from build123d import *

# Parameters (mm, degrees)
SKETCH1_R               = 2.5
EXTRUDE1_DEPTH          = 277.5
CUT_EXTRUDE1_DEPTH      = 556.900170894
CUT_EXTRUDE1_DEPTH_BACK = 556.900170894
SKETCH2_W               = 3.3
SKETCH2_H               = 11.078679656
SKETCH3_W               = 21.963498752
SKETCH3_H               = 21.444138823
CUT_EXTRUDE2_DEPTH      = 20


with BuildPart() as part:
    # Sketch1 → Extrude1 (new, symmetric)
    with BuildSketch(Plane.XY):
        with BuildLine():
            Line((0, 3.9), (-2.010912703, 3.9))
            ThreePointArc((-2.010912703, 3.9), (-2.776279568, 4.052240935), (-3.425126266, 4.485786438))
            Line((-3.425126266, 4.485786438), (-5.539339828, 6.6))
            Line((-5.539339828, 6.6), (-5.539339828, 8.2))
            Line((-5.539339828, 8.2), (-3.1, 8.2))
            Line((-3.1, 8.2), (-3.1, 9.5))
            Line((-3.1, 9.5), (-3.4, 9.5))
            ThreePointArc((-3.4, 9.5), (-3.541421356, 9.558578644), (-3.6, 9.7))
            Line((-3.6, 9.7), (-3.6, 10))
            Line((-3.6, 10), (-8.5, 10))
            Line((-8.5, 10), (-11.5, 10))
            Line((-11.5, 10), (-16.4, 10))
            Line((-16.4, 10), (-16.4, 9.7))
            ThreePointArc((-16.4, 9.7), (-16.458578644, 9.558578644), (-16.6, 9.5))
            Line((-16.6, 9.5), (-16.9, 9.5))
            Line((-16.9, 9.5), (-16.9, 8.2))
            Line((-16.9, 8.2), (-14.460660172, 8.2))
            Line((-14.460660172, 8.2), (-14.460660172, 6.6))
            Line((-14.460660172, 6.6), (-16.574873734, 4.485786438))
            ThreePointArc((-16.574873734, 4.485786438), (-17.223720432, 4.052240935), (-17.989087297, 3.9))
            Line((-17.989087297, 3.9), (-20, 3.9))
            Line((-20, 3.9), (-22.010912703, 3.9))
            ThreePointArc((-22.010912703, 3.9), (-22.776279568, 4.052240935), (-23.425126266, 4.485786438))
            Line((-23.425126266, 4.485786438), (-25.539339828, 6.6))
            Line((-25.539339828, 6.6), (-25.539339828, 8.2))
            Line((-25.539339828, 8.2), (-23.1, 8.2))
            Line((-23.1, 8.2), (-23.1, 9.5))
            Line((-23.1, 9.5), (-23.4, 9.5))
            ThreePointArc((-23.4, 9.5), (-23.541421356, 9.558578644), (-23.6, 9.7))
            Line((-23.6, 9.7), (-23.6, 10))
            Line((-23.6, 10), (-28.5, 10))
            ThreePointArc((-28.5, 10), (-29.560660172, 9.560660172), (-30, 8.5))
            Line((-30, 8.5), (-30, 3.6))
            Line((-30, 3.6), (-29.7, 3.6))
            ThreePointArc((-29.7, 3.6), (-29.558578644, 3.541421356), (-29.5, 3.4))
            Line((-29.5, 3.4), (-29.5, 3.1))
            Line((-29.5, 3.1), (-28.2, 3.1))
            Line((-28.2, 3.1), (-28.2, 5.539339828))
            Line((-28.2, 5.539339828), (-26.6, 5.539339828))
            Line((-26.6, 5.539339828), (-24.485786438, 3.425126266))
            ThreePointArc((-24.485786438, 3.425126266), (-24.052240935, 2.776279568), (-23.9, 2.010912703))
            Line((-23.9, 2.010912703), (-23.9, 0))
            Line((-23.9, 0), (-23.9, -2.010912703))
            ThreePointArc((-23.9, -2.010912703), (-24.052240935, -2.776279568), (-24.485786438, -3.425126266))
            Line((-24.485786438, -3.425126266), (-26.6, -5.539339828))
            Line((-26.6, -5.539339828), (-28.2, -5.539339828))
            Line((-28.2, -5.539339828), (-28.2, -3.1))
            Line((-28.2, -3.1), (-29.5, -3.1))
            Line((-29.5, -3.1), (-29.5, -3.4))
            ThreePointArc((-29.5, -3.4), (-29.558578644, -3.541421356), (-29.7, -3.6))
            Line((-29.7, -3.6), (-30, -3.6))
            Line((-30, -3.6), (-30, -8.5))
            ThreePointArc((-30, -8.5), (-29.560660172, -9.560660172), (-28.5, -10))
            Line((-28.5, -10), (-23.6, -10))
            Line((-23.6, -10), (-23.6, -9.7))
            ThreePointArc((-23.6, -9.7), (-23.541421356, -9.558578644), (-23.4, -9.5))
            Line((-23.4, -9.5), (-23.1, -9.5))
            Line((-23.1, -9.5), (-23.1, -8.2))
            Line((-23.1, -8.2), (-25.539339828, -8.2))
            Line((-25.539339828, -8.2), (-25.539339828, -6.6))
            Line((-25.539339828, -6.6), (-23.425126266, -4.485786438))
            ThreePointArc((-23.425126266, -4.485786438), (-22.776279568, -4.052240935), (-22.010912703, -3.9))
            Line((-22.010912703, -3.9), (-20, -3.9))
            Line((-20, -3.9), (-17.989087297, -3.9))
            ThreePointArc((-17.989087297, -3.9), (-17.223720432, -4.052240935), (-16.574873734, -4.485786438))
            Line((-16.574873734, -4.485786438), (-14.460660172, -6.6))
            Line((-14.460660172, -6.6), (-14.460660172, -8.2))
            Line((-14.460660172, -8.2), (-16.9, -8.2))
            Line((-16.9, -8.2), (-16.9, -9.5))
            Line((-16.9, -9.5), (-16.6, -9.5))
            ThreePointArc((-16.6, -9.5), (-16.458578644, -9.558578644), (-16.4, -9.7))
            Line((-16.4, -9.7), (-16.4, -10))
            Line((-16.4, -10), (-11.5, -10))
            Line((-11.5, -10), (-8.5, -10))
            Line((-8.5, -10), (-3.6, -10))
            Line((-3.6, -10), (-3.6, -9.7))
            ThreePointArc((-3.6, -9.7), (-3.541421356, -9.558578644), (-3.4, -9.5))
            Line((-3.4, -9.5), (-3.1, -9.5))
            Line((-3.1, -9.5), (-3.1, -8.2))
            Line((-3.1, -8.2), (-5.539339828, -8.2))
            Line((-5.539339828, -8.2), (-5.539339828, -6.6))
            Line((-5.539339828, -6.6), (-3.425126266, -4.485786438))
            ThreePointArc((-3.425126266, -4.485786438), (-2.776279568, -4.052240935), (-2.010912703, -3.9))
            Line((-2.010912703, -3.9), (0, -3.9))
            Line((0, -3.9), (2.010912703, -3.9))
            ThreePointArc((2.010912703, -3.9), (2.776279568, -4.052240935), (3.425126266, -4.485786438))
            Line((3.425126266, -4.485786438), (5.539339828, -6.6))
            Line((5.539339828, -6.6), (5.539339828, -8.2))
            Line((5.539339828, -8.2), (3.1, -8.2))
            Line((3.1, -8.2), (3.1, -9.5))
            Line((3.1, -9.5), (3.4, -9.5))
            ThreePointArc((3.4, -9.5), (3.541421356, -9.558578644), (3.6, -9.7))
            Line((3.6, -9.7), (3.6, -10))
            Line((3.6, -10), (8.5, -10))
            ThreePointArc((8.5, -10), (9.560660172, -9.560660172), (10, -8.5))
            Line((10, -8.5), (10, -3.6))
            Line((10, -3.6), (9.7, -3.6))
            ThreePointArc((9.7, -3.6), (9.558578644, -3.541421356), (9.5, -3.4))
            Line((9.5, -3.4), (9.5, -3.1))
            Line((9.5, -3.1), (8.2, -3.1))
            Line((8.2, -3.1), (8.2, -5.539339828))
            Line((8.2, -5.539339828), (6.6, -5.539339828))
            Line((6.6, -5.539339828), (4.485786438, -3.425126266))
            ThreePointArc((4.485786438, -3.425126266), (4.052240935, -2.776279568), (3.9, -2.010912703))
            Line((3.9, -2.010912703), (3.9, 0))
            Line((3.9, 0), (3.9, 2.010912703))
            ThreePointArc((3.9, 2.010912703), (4.052240935, 2.776279568), (4.485786438, 3.425126266))
            Line((4.485786438, 3.425126266), (6.6, 5.539339828))
            Line((6.6, 5.539339828), (8.2, 5.539339828))
            Line((8.2, 5.539339828), (8.2, 3.1))
            Line((8.2, 3.1), (9.5, 3.1))
            Line((9.5, 3.1), (9.5, 3.4))
            ThreePointArc((9.5, 3.4), (9.558578644, 3.541421356), (9.7, 3.6))
            Line((9.7, 3.6), (10, 3.6))
            Line((10, 3.6), (10, 8.5))
            ThreePointArc((10, 8.5), (9.560660172, 9.560660172), (8.5, 10))
            Line((8.5, 10), (3.6, 10))
            Line((3.6, 10), (3.6, 9.7))
            ThreePointArc((3.6, 9.7), (3.541421356, 9.558578644), (3.4, 9.5))
            Line((3.4, 9.5), (3.1, 9.5))
            Line((3.1, 9.5), (3.1, 8.2))
            Line((3.1, 8.2), (5.539339828, 8.2))
            Line((5.539339828, 8.2), (5.539339828, 6.6))
            Line((5.539339828, 6.6), (3.425126266, 4.485786438))
            ThreePointArc((3.425126266, 4.485786438), (2.776279568, 4.052240935), (2.010912703, 3.9))
            Line((2.010912703, 3.9), (0, 3.9))
        make_face()
        Circle(SKETCH1_R, mode=Mode.SUBTRACT)
        with Locations(Location((-20, 0, 0), (0, 0, 180))):
            Circle(SKETCH1_R, mode=Mode.SUBTRACT)
        with BuildLine():
            Line((-9.7, 3.6), (-10, 3.6))
            ThreePointArc((-10, 3.6), (-10.141421356, 3.541421356), (-10.2, 3.4))
            Line((-10.2, 3.4), (-10.2, 3.1))
            Line((-10.2, 3.1), (-11.5, 3.1))
            Line((-11.5, 3.1), (-11.5, 5.539339828))
            Line((-11.5, 5.539339828), (-13.1, 5.539339828))
            Line((-13.1, 5.539339828), (-15.214213562, 3.425126266))
            ThreePointArc((-15.214213562, 3.425126266), (-15.647759065, 2.776279568), (-15.8, 2.010912703))
            Line((-15.8, 2.010912703), (-15.8, 0))
            Line((-15.8, 0), (-15.8, -2.010912703))
            ThreePointArc((-15.8, -2.010912703), (-15.647759065, -2.776279568), (-15.214213562, -3.425126266))
            Line((-15.214213562, -3.425126266), (-13.1, -5.539339828))
            Line((-13.1, -5.539339828), (-11.5, -5.539339828))
            Line((-11.5, -5.539339828), (-11.5, -3.1))
            Line((-11.5, -3.1), (-10.2, -3.1))
            Line((-10.2, -3.1), (-10.2, -3.4))
            ThreePointArc((-10.2, -3.4), (-10.141421356, -3.541421356), (-10, -3.6))
            Line((-10, -3.6), (-9.7, -3.6))
            ThreePointArc((-9.7, -3.6), (-9.558578644, -3.541421356), (-9.5, -3.4))
            Line((-9.5, -3.4), (-9.5, -3.1))
            Line((-9.5, -3.1), (-8.2, -3.1))
            Line((-8.2, -3.1), (-8.2, -5.539339828))
            Line((-8.2, -5.539339828), (-6.6, -5.539339828))
            Line((-6.6, -5.539339828), (-4.485786438, -3.425126266))
            ThreePointArc((-4.485786438, -3.425126266), (-4.052240935, -2.776279568), (-3.9, -2.010912703))
            Line((-3.9, -2.010912703), (-3.9, 0))
            Line((-3.9, 0), (-3.9, 2.010912703))
            ThreePointArc((-3.9, 2.010912703), (-4.052240935, 2.776279568), (-4.485786438, 3.425126266))
            Line((-4.485786438, 3.425126266), (-6.6, 5.539339828))
            Line((-6.6, 5.539339828), (-8.2, 5.539339828))
            Line((-8.2, 5.539339828), (-8.2, 3.1))
            Line((-8.2, 3.1), (-9.5, 3.1))
            Line((-9.5, 3.1), (-9.5, 3.4))
            ThreePointArc((-9.5, 3.4), (-9.558578644, 3.541421356), (-9.7, 3.6))
        make_face(mode=Mode.SUBTRACT)
    extrude(amount=EXTRUDE1_DEPTH, both=True)

    # Sketch2 → Cut-Extrude1 (cut, two sides: drawn at the far end of the back side and taken through both)
    with BuildSketch(Plane.XY.offset(277.5).offset(-CUT_EXTRUDE1_DEPTH_BACK)):
        with Locations((-9.85, 0)):
            Rectangle(SKETCH2_W, SKETCH2_H)
    extrude(amount=CUT_EXTRUDE1_DEPTH + CUT_EXTRUDE1_DEPTH_BACK, mode=Mode.SUBTRACT)

    # Sketch3 → Cut-Extrude2 (cut)
    with BuildSketch(Plane.XY.offset(277.5)):
        with Locations((-20.981749376, 0.722069412)):
            Rectangle(SKETCH3_W, SKETCH3_H)
    cut_extrude2 = extrude(amount=-CUT_EXTRUDE2_DEPTH, mode=Mode.SUBTRACT)

    # Mirror1: Cut-Extrude2 across plane
    add(cut_extrude2.mirror(Plane.XY), mode=Mode.SUBTRACT)


solid = part.part
Verification items for the finished model (mm, model axes). A direction names the side the tool comes from. Round coordinates to 2 decimals unless told otherwise and drop trailing zeros. Use a Markdown table: item, result. Add a question column.
1. Thickness scan on probe 1 along X at (y, z) = (-7.5, 211); probe 2 along X at (y, z) = (-0.25, 221); probe 3 along X at (y, z) = (-0.5, -68). Record the ranges inside material, lowest first. Write a range as [from, to].
2. Gauge pin test, flat ends, axial feed: pin 1 (1.5 mm diameter, centred on x = -19.5, y = -1, fed in from +Z); pin 2 (6 mm diameter, centred on x = -20, y = -2.5, fed in from +Z); pin 3 (1 mm diameter, centred on x = 1.5, z = -131, fed in from -Y). Record the tip position at first contact, or that the pin passes through.
3. Access from +Z, -Z, +X, -X, +Y, -Y to the whole of each face (thin tool, end or side, straight path). Record for faces 1 (the face through (2, 2, 277.5)), 2 (the face through (-22, 2, 257.5)), 3 (the face through (-22, 2, -257.5)).
4. Section check A-A, the plane z = 195. Give the number of separate pieces and of enclosed holes in the cut face, plus the area to 3 significant figures.
Checks:
| question | item | result |
|---|---|---|
| 1 | probe 1 | x = [-30, -25.54], [-14.46, -5.54], [5.54, 10] |
| 1 | probe 2 | x = [-23.9, -22.49], [-17.51, -15.8], [-3.9, -2.49], [2.49, 3.9] |
| 1 | probe 3 | x = [-23.9, -22.45], [-17.55, -15.8], [-3.9, -2.45], [2.45, 3.9] |
| 2 | pin 1 | passes through |
| 2 | pin 2 | stops at z = 257.5 |
| 2 | pin 3 | stops at y = -3.9 |
| 3 | face 1 | +Z, +X, -X, +Y, -Y |
| 3 | face 2 | +Z, -X, +Y, -Y |
| 3 | face 3 | -Z, -X, +Y, -Y |
| 4 | separate pieces | 1 |
| 4 | enclosed holes | 3 |
| 4 | area | 331 mm^2 |
